Autodesk Inventor part; units mm, degrees
ref_plane "YZ Plane" through (0, 0, 0) normal (1, 0, 0) x (0, 1, 0)
ref_plane "XZ Plane" through (0, 0, 0) normal (0, 1, 0) x (-1, 0, 0)
ref_plane "XY Plane" through (0, 0, 0) normal (0, 0, 1) x (1, 0, 0)
sketch "Sketch1" plane through (0, 0, 0) normal (1, 0, 0) x (0, 1, 0)
  line L0 (-19.8, 28) -> (19.8, 28)
  line L1 (19.8, 28) -> (19.8, -28)
  line L2 (19.8, -28) -> (-19.8, -28)
  line L3 (-19.8, -28) -> (-19.8, 28)
  line L4 (-19.8, 28) -> (19.8, -28) construction
  line L5 (19.8, 28) -> (-19.8, -28) construction
  point P0 (0, 0)
  dimension "d0" = 39.6
  dimension "d1" = 56
extrude "Extrusion1" add sketch "Sketch1" along normal blind 40
sketch "Sketch2" plane through (0, -19.8, 28) normal (0, 0, 1) x (1, 0, 0)
  line L0 (7.8, 0) -> (32.2, 0)
  line L1 (32.2, 0) -> (32.2, 31.8)
  line L2 (32.2, 31.8) -> (7.8, 31.8)
  line L3 (7.8, 31.8) -> (7.8, 0)
  line L4 (0, 0) -> (40, 0)
  line L5 (40, 39.6) -> (40, 0)
  dimension "d4" = 24.4
  dimension "d5" = 31.8
  dimension "d6" = 7.8
extrude "Extrusion2" cut sketch "Sketch2" against normal blind 64
sketch "Sketch3" plane through (32.2, -19.8, 28) normal (-1, 0, 0) x (0, 0, 1)
  circle A0 centre (-12, 3.8502) radius 2.3
  circle A1 centre (-28, 3.8502) radius 2.3
  line L0 (0, 31.8) -> (0, 0)
  point P0 (-28, 19.8)
  dimension "d9" = 4.6
  dimension "d10" = 4.6
  dimension "d11" = 16
  dimension "d12" = 12
extrude "Extrusion3" add sketch "Sketch3" along normal blind 26
sketch "Sketch4" plane through (7.8, -19.8, 28) normal (1, 0, 0) x (0, 0, -1)
  line L0 (56, 0) -> (0, 0)
  line L1 (56, 0) -> (32, 0)
  line L2 (32, 0) -> (32, 8)
  line L3 (32, 8) -> (56, 8)
  line L4 (56, 8) -> (56, 0)
  point P0 (28, 19.8)
  point P1 (32, 0)
  dimension "d15" = 24
  dimension "d16" = 8
extrude "Extrusion4" add sketch "Sketch4" along normal blind 26
sketch "Sketch14" plane through (0, 19.8, 28) normal (0, 1, 0) x (1, 0, 0)
  line L0 (20, 0) -> (20, 56)
  point P0 (0, 28)
sketch "Sketch15" plane through (0, -19.8, -28) normal (0, -1, 0) x (1, 0, 0)
  line L0 (40, 0) -> (40, 56)
  line L1 (0, 0) -> (40, 0)
  line L2 (0, 56) -> (40, 56)
  line L3 (0, 0) -> (0, 56)
  point P0 (0, 28)
extrude "Extrusion7" add sketch "Sketch15" along normal blind 24
sketch "Sketch16" plane through (0, 19.8, 28) normal (0, 0, 1) x (1, 0, 0)
  line L0 (8, -47.6) -> (32, -47.6)
  line L1 (32, -47.6) -> (32, -55.6)
  line L2 (32, -55.6) -> (8, -55.6)
  line L3 (8, -55.6) -> (8, -47.6)
  line L4 (40, -63.6) -> (0, -63.6)
  line L5 (0, 0) -> (0, -63.6)
  line L6 (16, -55.6) -> (24, -55.6)
  line L7 (24, -55.6) -> (24, -63.6)
  line L8 (24, -63.6) -> (16, -63.6)
  line L9 (16, -63.6) -> (16, -55.6)
  point P0 (0, -19.8)
  dimension "d37" = 24
  dimension "d38" = 8
  dimension "d39" = 8
  dimension "d40" = 8
  dimension "d41" = 8
  dimension "d42" = 8
  dimension "d43" = 16
extrude "Extrusion8" cut sketch "Sketch16" against normal through all
chamfer "Chamfer1" distance 8 angle 45 2 edges at (40, -43.8, 0) (0, -43.8, 0)
chamfer "Chamfer2" distance 8 angle 45 2 edges at (16, -35.8, 0) (24, -35.8, 0)
properties part number "MotorHolder_X"
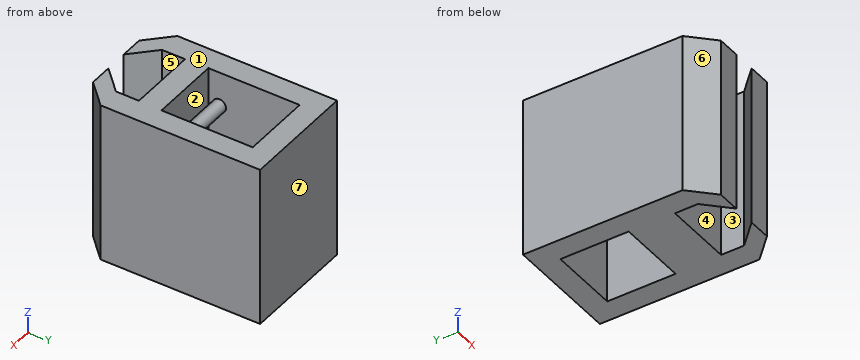
The model under review builds one solid part; all positions refer to its coordinate system, in mm. Face numbers are marked on the shaded views. A direction names the side the tool comes from. Round coordinates to 2 decimals unless told otherwise and drop trailing zeros. Write each loop counter-clockwise with the first axis right and the second up, starting at its lowest first coordinate (ties: lowest second). Pieces come first, ordered by that corner, then holes.
(1) We need section B-B on y = 10.5. Give the boundary of the cut face in (x, z), and give its area (3 significant figures).
(2) Mouldability with a two-part tool opening along X and no side actions: class the marked faces 4, 5, 6 and 7 as +X half, -X half, draft (parallel to the pull), parting line (faces both ways), or undercut.
(3) Wall thickness on L1, parallel to X at y = 11, z = -13; L2, parallel to X at y = -35, z = -14; L3, parallel to Y at x = 31, z = 2: over which ranges is each line inside the solid? List them lowest first.
(4) Machinability: for the marked faces 1, 2 and 3, which of the approach directions +Z, -Z, +X, -X, +Y, -Y give a long, thin tool a straight path to every point of the face, cutting with its end or side? Answer none if there is none.
(5) Insertion check: pin 1 (4 mm diameter, centred on x = 21.5, z = 13.5, fed in from -Y); pin 2 (2.5 mm diameter, centred on x = 22, y = -14, fed in from +Z). Each pin has a flat end and moves straight along its axis. Give the tip position at first contact, or say it passes through.
(6) We need section A-A on z = 0. Give the number of separate pieces and of enclosed holes in the cut face, and give its area (3 significant figures).
(7) We need section D-D on x = 11. Give the boundary of the cut face in (y, z), and give its area (3 significant figures).
Findings below:
1. outline: (0, -28) - (7.8, -28) - (7.8, 28) - (0, 28) - close; (32.2, -28) - (40, -28) - (40, 28) - (32.2, 28) - close
1. area: 874 mm2
2. face 4: undercut
2. face 5: undercut
2. face 6: -X half
2. face 7: draft
3. L1: x = 0 to 7.8, 32.2 to 40
3. L2: x = 0 to 8, 32 to 40
3. L3: y = -43.8 to -36.8, -27.8 to -19.8, -17.09 to -14.81, 12 to 19.8
4. face 1: +Z, +X, -X, +Y, -Y
4. face 2: +Z
4. face 3: +Z, -Z
5. pin 1: stops at y = -27.8
5. pin 2: stops at z = 18.19
6. separate pieces: 1
6. enclosed holes: 2
6. area: 1,500 mm2
7. outline: (-43.8, -28) - (-38.8, -28) - (-38.8, 28) - (-43.8, 28) - close; (-27.8, -28) - (-11.8, -28) - (-11.8, -4) - (-19.8, -4) - (-19.8, 28) - (-27.8, 28) - close; circle Ø4.6 at (-15.95, 0); circle Ø4.6 at (-15.95, 16); (12, -28) - (19.8, -28) - (19.8, 28) - (12, 28) - close
7. area: 1,390 mm2
